Check sheet for the modelled part. Datum: model origin and axes. Units: mm. Face numbers are marked on the shaded views. Round coordinates to 2 decimals unless told otherwise and drop trailing zeros. Loops run counter-clockwise (first coordinate to the right, second up) from the corner with the lowest first, then second, coordinate; pieces in that order, holes last. Notation, with made-up numbers: (33.5, 65) -> (61.5, 65) arc R28 cw to (61.5, 101) -> close; hole circle Ø7 at (30.5, -10). An arc over 180 degrees is marked (long way). Use one line per item in the form item = value. Start each with the question number.
(1) Go/stop test with flat-tipped pins: pin 1 (6 mm diameter, centred on x = 63.5, y = -26.5, fed in from +Z); pin 2 (8 mm diameter, centred on y = -5.5, z = 14.5, fed in from -X); pin 3 (6 mm diameter, centred on y = -15, z = 0.5, fed in from -X). Record where each tip stops, or that it passes through.
(2) Sectioned sample at B-B (y = -6). Record the cut outline in (x, z).
(3) Material ranges on probe 1 along Z at (x, y) = (0, -33.5); probe 2 along Y at (x, z) = (76, -2); probe 3 along Z at (x, y) = (90, -10), recorded low to high. Write a range as [from, to].
(4) Sectioned sample at D-D (z = 2.5). State how many separate pieces and enclosed holes the cut face has, and give its area (3 significant figures).
(5) Draft check along X on the marked faces 1, 2 and 3. Enter one of: released by +X, released by -X, zero draft, split by the parting line, or undercut.
(6) Sectioned sample at A-A (x = 0). Record the cut outline in (y, z), and give its area (3 significant figures).
(7) Sectioned sample at C-C (y = -33.5). Record the cut outline in (x, z), and give its area (3 significant figures).
from build123d import *

# Parameters (mm, degrees)
F0_R     = 10
F1_DEPTH = 25
F2_DEPTH = 50
F3_SIZE  = 3
F4_SIZE  = 1


with BuildPart() as f1:
    # F0 (on Front) → F1 (new body)
    with BuildSketch(Plane.XZ):
        with BuildLine():
            ThreePointArc((2.083333, -24.913043), (18.399502, -16.92508), (25, 0))
            ThreePointArc((25, 0), (18.399502, 16.92508), (2.083333, 24.913043))
            ThreePointArc((2.083333, 24.913043), (-25, 0), (2.083333, -24.913043))
        make_face()
        Circle(F0_R, mode=Mode.SUBTRACT)
        with BuildLine():
            ThreePointArc((2.083333, 24.913043), (18.399502, 16.92508), (25, 0))
            ThreePointArc((25, 0), (18.399502, -16.92508), (2.083333, -24.913043))
            Line((2.083333, -24.913043), (91.458333, -17.43913))
            ThreePointArc((91.458333, -17.43913), (72.5, 0), (91.458333, 17.43913))
            Line((91.458333, 17.43913), (2.083333, 24.913043))
        make_face()
        with BuildLine():
            ThreePointArc((107.5, 0), (102.879651, 11.847556), (91.458333, 17.43913))
            ThreePointArc((91.458333, 17.43913), (72.5, 0), (91.458333, -17.43913))
            ThreePointArc((91.458333, -17.43913), (102.879651, -11.847556), (107.5, 0))
        make_face()
        with Locations((90, 0)):
            Circle(F0_R, mode=Mode.SUBTRACT)
    extrude(amount=F1_DEPTH)

    # F0 (on Front) → F2 (join)
    with BuildSketch(Plane.XZ):
        with BuildLine():
            ThreePointArc((2.083333, -24.913043), (18.399502, -16.92508), (25, 0))
            ThreePointArc((25, 0), (18.399502, 16.92508), (2.083333, 24.913043))
            ThreePointArc((2.083333, 24.913043), (-25, 0), (2.083333, -24.913043))
        make_face()
        Circle(F0_R, mode=Mode.SUBTRACT)
    extrude(amount=F2_DEPTH)

    # F3
    f3_edges = [f1.edges().sort_by_distance(p)[0] for p in [
        (-2.083333, -50, 24.913043),
        (-10, -50, 0),
        (80, -25, 0),
    ]]
    chamfer(f3_edges, length=F3_SIZE)

    # F4
    f4_edges = [f1.edges().sort_by_distance(p)[0] for p in [
        (-25, 0, 0),
        (46.770833, 0, -21.176087),
        (107.5, 0, 0),
        (46.770833, 0, 21.176087),
        (-10, 0, 0),
        (80, 0, 0),
    ]]
    chamfer(f4_edges, length=F4_SIZE)


solid = f1.part
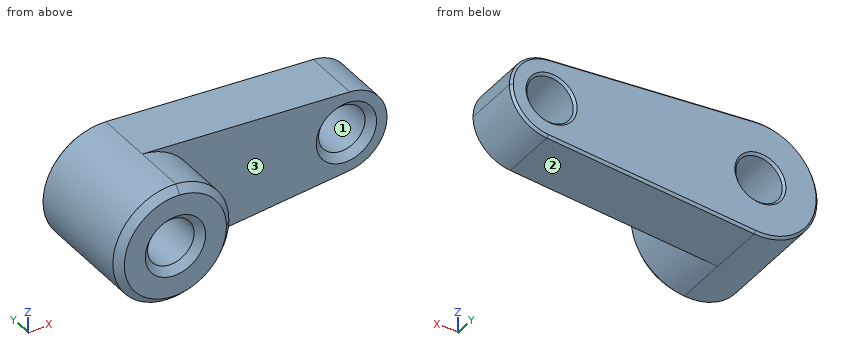
Checks:
q1.pin_1 = 19.99
q1.pin_2 = -22.69
q1.pin_3 = -25
q2.outline = (2.08, -24.91) -> (91.46, -17.44) arc R17.5 ccw to (91.46, 17.44) -> (2.08, 24.91) arc R25 ccw (long way) to start; hole circle Ø20 at (0, 0); hole circle Ø20 at (90, 0)
q3.probe_1 = [-25, -10], [10, 25]
q3.probe_2 = [-25, 0]
q3.probe_3 = [-17.56, -10], [10, 17.56]
q4.separate_pieces = 3
q4.enclosed_holes = 0
q4.area = 3,070 mm2
q5.face_1 = undercut
q5.face_2 = released by +X
q5.face_3 = zero draft
q6.outline = (-50, -22) -> (-47, -25) -> (-1, -25) -> (0, -24) -> (0, -11) -> (-1, -10) -> (-47, -10) -> (-50, -13) -> close; (-50, 13) -> (-47, 10) -> (-1, 10) -> (0, 11) -> (0, 24) -> (-1, 25) -> (-47, 25) -> (-50, 22) -> close
q6.area = 1,480 mm2
q7.outline = (2.08, -24.91) arc R25 ccw to (25, 0) arc R25 ccw to (2.08, 24.91) arc R25 ccw (long way) to start; hole circle Ø20 at (0, 0)
q7.area = 1,650 mm2
